For this review, take the finished solid that the model builds, in its own axes (mm). Coordinates: 2 decimals unless noted, no trailing zeros. Write each loop counter-clockwise with the first axis right and the second up, starting at its lowest first coordinate (ties: lowest second). Pieces come first, ordered by that corner, then holes.
```python
from build123d import *

# Parameters (mm, degrees)
CROQUIS1_R              = 100
SALIENTE_EXTRUIR1_DEPTH = 3
CROQUIS3_R              = 110
CORTAR_EXTRUIR1_DEPTH   = 3
REDONDEO1_R             = 10
CROQUIS4_W              = 25
CROQUIS4_H              = 100
CORTAR_EXTRUIR2_DEPTH   = 142.453172607


with BuildPart() as part:
    # Croquis1 → Saliente-Extruir1 (new body)
    with BuildSketch(Plane.XY):
        Circle(CROQUIS1_R)
    extrude(amount=SALIENTE_EXTRUIR1_DEPTH)

    # Croquis3 → Cortar-Extruir1 (cut)
    with BuildSketch(Plane.XY.offset(3)):
        with Locations((190, 0)):
            Circle(CROQUIS3_R)
    extrude(amount=-CORTAR_EXTRUIR1_DEPTH, mode=Mode.SUBTRACT)

    # Redondeo1
    redondeo1_edges = [part.edges().sort_by_distance(p)[0] for p in [
        (89.473684211, -44.659375654, 1.5),
        (89.473684211, 44.659375654, 1.5),
    ]]
    fillet(redondeo1_edges, radius=REDONDEO1_R)

    # Croquis4 → Cortar-Extruir2 (cut, through all)
    with BuildSketch(Plane(origin=(0, 0, 0), x_dir=(-1, 0, 0), z_dir=(0, 0, -1))):
        with Locations((52.5, 0)):
            Rectangle(CROQUIS4_W, CROQUIS4_H)
    extrude(amount=-CORTAR_EXTRUIR2_DEPTH, mode=Mode.SUBTRACT)


solid = part.part
```
Q1. Draft analysis for pull direction Y (two halves, no side actions). For faces 1 (the cylindrical face through (-99.932, 3.679, 1.479)), 2 (the flat face through (-7, 1, 3)), 3 (the cylindrical face through (80, 0.6, 1.5)), state which applies: +Y half, -Y half, draft (parallel to the pull), parting line (faces both ways), or undercut.
Ans:
face 1: parting line
face 2: draft
face 3: undercut
Q2. Add section C-C (x = 33.5). State the section outline as (y, z) points, then the cut area to 3 significant figures.
Ans:
outline: (-94.22, 0) - (94.22, 0) - (94.22, 3) - (-94.22, 3) - close
area: 565 mm2
Q3. For probe 1 along X at (y, z) = (9.5, 2.3); probe 2 along X at (y, z) = (-29, 1.5); probe 3 along Y at (x, z) = (-3, 2.1), list the stretches that pass through material, from the lowest coordinate up.
Ans:
probe 1: x = -99.55 to -65, -40 to 80.41
probe 2: x = -95.7 to -65, -40 to 83.89
probe 3: y = -99.95 to 99.95
Q4. Add section A-A (y = 0). State the section outline as (x, z) points.
Ans:
outline: (-100, 0) - (-65, 0) - (-65, 3) - (-100, 3) - close; (-40, 0) - (80, 0) - (80, 3) - (-40, 3) - close
Q5. Add section B-B (y = 34). State the section outline as (x, z) points, then the cut area to 3 significant figures.
Ans:
outline: (-94.04, 0) - (-65, 0) - (-65, 3) - (-94.04, 3) - close; (-40, 0) - (85.39, 0) - (85.39, 3) - (-40, 3) - close
area: 463 mm2
Q6. Clearance check with a flat-ended pin moving along its axis: pin 1 Ø1.5 at (y, z) = (9.5, 1.5) entering from +X. State where the tip first meets the part, or that it passes through.
Ans:
pin 1: stops at x = 80.48
Q7. Add section D-D (y = -61). State the section outline as (x, z) points, then the cut area to 3 significant figures.
Ans:
outline: (-79.24, 0) - (79.24, 0) - (79.24, 3) - (-79.24, 3) - close
area: 475 mm2
